```python
from build123d import *

# Parameters (mm, degrees)
SKETCH1_W           = 184
SKETCH1_H           = 86
BOSS_EXTRUDE1_DEPTH = 6
SKETCH2_W           = 6
SKETCH2_H           = 6
BOSS_EXTRUDE2_DEPTH = 6
SKETCH3_W           = 100
SKETCH3_H           = 30
CUT_EXTRUDE1_DEPTH  = 6


with BuildPart() as part:
    # Sketch1 → Boss-Extrude1 (new body)
    with BuildSketch(Plane.XY):
        with Locations((0, 43)):
            Rectangle(SKETCH1_W, SKETCH1_H)
    extrude(amount=BOSS_EXTRUDE1_DEPTH)

    # Sketch2 → Boss-Extrude2 (add)
    with BuildSketch(Plane.XY):
        with Locations((-77, -3)):
            Rectangle(SKETCH2_W, SKETCH2_H)
        with Locations((-26, -3)):
            Rectangle(SKETCH2_W, SKETCH2_H)
        with Locations((26, -3)):
            Rectangle(SKETCH2_W, SKETCH2_H)
        with Locations((77, -3)):
            Rectangle(SKETCH2_W, SKETCH2_H)
        with Locations((-75, 89)):
            Rectangle(SKETCH2_W, SKETCH2_H)
        with Locations((-24, 89)):
            Rectangle(SKETCH2_W, SKETCH2_H)
        with Locations((24, 89)):
            Rectangle(SKETCH2_W, SKETCH2_H)
        with Locations((75, 89)):
            Rectangle(SKETCH2_W, SKETCH2_H)
    extrude(amount=BOSS_EXTRUDE2_DEPTH)

    # Sketch3 → Cut-Extrude1 (cut)
    with BuildSketch(Plane.XY.offset(6)):
        with Locations((0, 43)):
            Rectangle(SKETCH3_W, SKETCH3_H)
    extrude(amount=-CUT_EXTRUDE1_DEPTH, mode=Mode.SUBTRACT)


solid = part.part
```
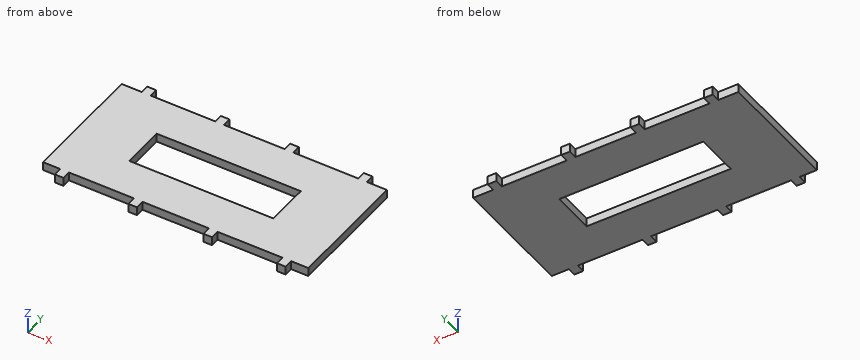
The listing builds one solid part. Answer for the finished solid, in the listing's coordinates (mm). Round coordinates to 2 decimals unless told otherwise and drop trailing zeros. Write each loop counter-clockwise with the first axis right and the second up, starting at its lowest first coordinate (ties: lowest second). Pieces come first, ordered by that corner, then holes. Notation, with made-up numbers: (12.25, -34) -> (68.25, -34) arc R8 cw to (68.25, -25) -> close; hole circle Ø1 at (19.5, -3.5). An arc over 180 degrees is marked (long way). Answer as a JSON object with one key per item and string values. Group by question number.
Q1. Section A-A (y = 38) is taken. Write down the section's boundary in (x, z).
Q2. Straight lines are drawn through the part: line 1 along X through (y, z) = (55, 3.25); line 2 along Y through (x, z) = (-14.5, 2); line 3 along Y through (x, z) = (28, 5.6). For each, find the intervals that lie inside material, in ascending order.
Q3. Each of these flat-tipped pins is pushed along its axis until it touches: pin 1 Ø3 at (y, z) = (-2.5, 3) entering from +X; pin 2 Ø3 at (x, z) = (-1.5, 3.5) entering from +Y; pin 3 Ø1.8 at (y, z) = (88, 4) entering from +X. Where does it stop, or does it pass through?
Q4. Section B-B (x = -42.5) is taken. Write down the section's boundary in (y, z).
Check values:
{
 "1": {"outline": "(-92, 0) -> (-50, 0) -> (-50, 6) -> (-92, 6) -> close; (50, 0) -> (92, 0) -> (92, 6) -> (50, 6) -> close"},
 "2": {"line 1": "-92 to -50, 50 to 92", "line 2": "0 to 28, 58 to 86", "line 3": "-6 to 28, 58 to 86"},
 "3": {"pin 1": "x = 80", "pin 2": "y = 86", "pin 3": "x = 78"},
 "4": {"outline": "(0, 0) -> (28, 0) -> (28, 6) -> (0, 6) -> close; (58, 0) -> (86, 0) -> (86, 6) -> (58, 6) -> close"}
}
